from build123d import *

# Parameters (mm, degrees)
F0_R     = 5.55625
F1_DEPTH = 25


# Not quite as in the source:
# - a feature names something its author has since deleted; it is built from what else it names


with BuildPart() as f1:
    # F0 (on Top) → F1 (new body)
    with BuildSketch(Plane.XY):
        with BuildLine():
            ThreePointArc((-69.0590284919, -1), (-69.0147699554, -0.5008703332), (-69, 0))
            ThreePointArc((-69, 0), (-69.0147699554, 0.5008703332), (-69.0590284919, 1))
            ThreePointArc((-69.0590284919, 1), (-69.6284732517, 3.2076575021), (-70.7642342114, 5.184540408))
            ThreePointArc((-70.7642342114, 5.184540408), (-86, 0), (-70.7642342114, -5.184540408))
            ThreePointArc((-70.7642342114, -5.184540408), (-69.6284732517, -3.2076575021), (-69.0590284919, -1))
        make_face()
        with Locations((-77.5, 0)):
            Circle(F0_R, mode=Mode.SUBTRACT)
        with BuildLine():
            ThreePointArc((-70.7642342114, 5.184540408), (-69.6284732517, 3.2076575021), (-69.0590284919, 1))
            Line((-69.0590284919, 1), (-64.4374042749, 1))
            add(Edge.make_bspline(
                [(-64.4374042749, 1), (-67.7107125521, 1), (-68.7326164375, 2.5450583285), (-70.7642342114, 5.184540408)],
                knots=[0, 0, 0, 0, 7.58545684, 7.58545684, 7.58545684, 7.58545684], degree=3))
        make_face()
        with BuildLine():
            Line((-64.4374042749, -1), (-69.0590284919, -1))
            ThreePointArc((-69.0590284919, -1), (-69.6284732517, -3.2076575021), (-70.7642342114, -5.184540408))
            add(Edge.make_bspline(
                [(-64.4374042749, -1), (-67.7107125521, -1), (-68.7326164375, -2.5450583285), (-70.7642342114, -5.184540408)],
                knots=[0, 0, 0, 0, 7.58545684, 7.58545684, 7.58545684, 7.58545684], degree=3))
        make_face()
        with BuildLine():
            ThreePointArc((-69.0590284919, 1), (-69.0147699554, 0.5008703332), (-69, 0))
            ThreePointArc((-69, 0), (-69.0147699554, -0.5008703332), (-69.0590284919, -1))
            Line((-69.0590284919, -1), (-64.4374042749, -1))
            Line((-64.4374042749, -1), (0, -1))
            Line((0, -1), (0, 1))
            Line((0, 1), (-64.4374042749, 1))
            Line((-64.4374042749, 1), (-69.0590284919, 1))
        make_face()
    extrude(amount=F1_DEPTH)


solid = f1.part
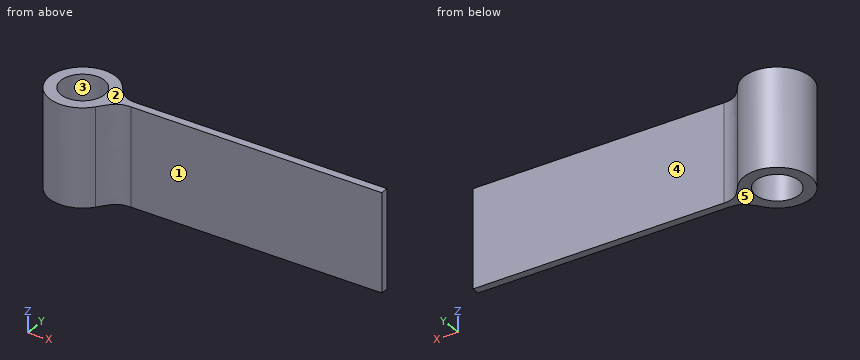
Can you work these out from the model? Positions are in its coordinate system, mm. Face numbers are marked on the shaded views. A direction names the side the tool comes from. Coordinates: 2 decimals unless noted, no trailing zeros. Loops run counter-clockwise (first coordinate to the right, second up) from the corner with the lowest first, then second, coordinate; pieces in that order, holes last. Notation, with made-up numbers: (13.5, 34) - (69.5, 34) arc R12 cw to (69.5, 48) - close; hole circle Ø6 at (-4, 79.5). An arc over 180 degrees is marked (long way). Answer as a JSON object with one key per item and string values. Group by question number.
Item 1: If we section it at B-B (y = 0): List the corners of the cut face in (x, z) for me, plus the area to 3 significant figures.
Item 2: For pin 1 (2 mm diameter, centred on x = -43, z = 18, fed in from -Y); pin 2 (8 mm diameter, centred on y = 1, z = 17.5, fed in from -X); pin 3 (7.5 mm diameter, centred on x = -40.5, z = 16, fed in from +Y); pin 4 (6 mm diameter, centred on x = -68.5, z = 20.5, fed in from -Y), each with a flat end and sliding along its axis, tell me the tip position at first contact or that it passes through.
Item 3: If we mould it in two halves opening along Y, with no side actions, what happens to the marked faces 1, 2 and 3? For each: released by +Y, released by -Y, zero draft, split by the parting line, or undercut.
Item 4: If we section it at C-C (x = -22): List the corners of the cut face in (y, z) for me, plus the area to 3 significant figures.
Item 5: If I drill on L1, parallel to Y at x = -77.5, z = 18.5; L2, parallel to Y at x = -41, z = 17.25; L3, parallel to X at y = -0.25, z = 1.75, over which ranges is the centre line in solid material (lowest first)? Write a range as from..to.
Item 6: On a 3-axis mill with a long thin cutter (end or side, diameter ignored), from which of +Z, -Z, +X, -X, +Y, -Y can I reach the whole of each face in a straight line? I mean the marked faces 4 and 5. Say none if no direction works.
Item 7: If we section it at A-A (x = -77.5): List the corners of the cut face in (y, z) for me.
Returned:
{
 "1": {"outline": "(-86, 0) - (-83.06, 0) - (-83.06, 25) - (-86, 25) - close; (-71.94, 0) - (0, 0) - (0, 25) - (-71.94, 25) - close", "area": "1,870 mm²"},
 "2": {"pin 1": "stops at y = -1", "pin 2": "stops at x = -86", "pin 3": "stops at y = 1", "pin 4": "stops at y = -6.02"},
 "3": {"face 1": "released by -Y", "face 2": "zero draft", "face 3": "undercut"},
 "4": {"outline": "(-1, 0) - (1, 0) - (1, 25) - (-1, 25) - close", "area": "50.0 mm²"},
 "5": {"L1": "y = -8.5..-5.56, 5.56..8.5", "L2": "y = -1..1", "L3": "x = -86..-83.05, -71.95..0"},
 "6": {"face 4": "+Z, -Z, +X, +Y", "face 5": "-Z, +X, -X, +Y, -Y"},
 "7": {"outline": "(-8.5, 0) - (-5.56, 0) - (-5.56, 25) - (-8.5, 25) - close; (5.56, 0) - (8.5, 0) - (8.5, 25) - (5.56, 25) - close"}
}
